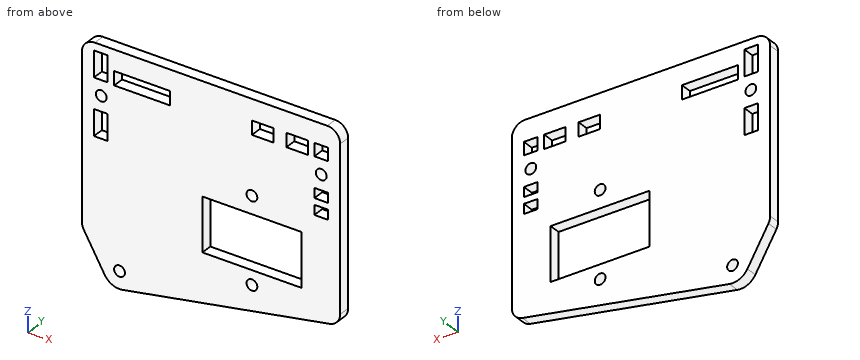
```python
from build123d import *
from build123d.topology import SkipClean

# Parameters (mm, degrees)
SKETCH1_R           = 1.25
SKETCH1_W           = 3.194492506
SKETCH1_H           = 3.000146449
SKETCH1_W_2         = 3.194434014
SKETCH1_H_2         = 6.000288014
SKETCH1_H_3         = 6.000224533
SKETCH1_W_3         = 4.990971694
SKETCH1_H_4         = 3.200091917
SKETCH1_W_4         = 4.991186163
SKETCH1_W_5         = 22.959409558
SKETCH1_H_5         = 12.40053533
BOSS_EXTRUDE1_DEPTH = 2.646066576


with BuildPart() as part:
    # Sketch1 → Boss-Extrude1 (new body)
    with SkipClean():  # the faces are left unmerged after this step: merging them gives an invalid solid
        with BuildSketch(Plane(origin=(0, 0, 0), x_dir=(1, 0, 0), z_dir=(0, 1, 0))):
            with BuildLine():
                Line((25.442900716, -27.532431428), (-28.456084878, -27.532431428))
                ThreePointArc((-28.456084878, -27.532431428), (-30.577373887, -26.653764751), (-31.456040564, -24.532475742))
                Line((-31.456040564, -24.532475742), (-31.456040564, 13.269326446))
                ThreePointArc((-31.456040564, 13.269326446), (-31.352979308, 14.049412081), (-31.050867612, 14.775968165))
                Line((-31.050867612, 14.775968165), (-26.174789125, 23.186205164))
                ThreePointArc((-26.174789125, 23.186205164), (-24.390968499, 24.809261571), (-21.997773241, 25.107497345))
                Line((-21.997773241, 25.107497345), (25.983223234, 16.219991273))
                ThreePointArc((25.983223234, 16.219991273), (27.743957441, 15.188191581), (28.437804204, 13.268980227))
                Line((28.437804204, 13.268980227), (28.437609204, -24.537738386))
                ThreePointArc((28.437609204, -24.537738386), (27.560473935, -26.65530708), (25.442900716, -27.532431428))
            make_face()
            with Locations(Location((-22.724218332, 21.185636807, 0), (0, 0, 270))):
                Circle(SKETCH1_R, mode=Mode.SUBTRACT)
            with Locations(Location((-26.963965218, -16.232064957, 0), (0, 0, 270))):
                Circle(SKETCH1_R, mode=Mode.SUBTRACT)
            with Locations(Location((7.974006473, 13.76898446, 0), (0, 0, 270))):
                Circle(SKETCH1_R, mode=Mode.SUBTRACT)
            with Locations(Location((7.974006472, -6.031549942, 0), (0, 0, 270))):
                Circle(SKETCH1_R, mode=Mode.SUBTRACT)
            with Locations(Location((24.045515173, -16.23206496, 0), (0, 0, 270))):
                Circle(SKETCH1_R, mode=Mode.SUBTRACT)
            Polygon((22.448181182, -10.478708085), (22.448181182, -10.484914569), (22.448181182, -12.731920553), (25.642673688, -12.731920553), (25.642673688, -10.478708085), align=None, mode=Mode.SUBTRACT)
            with Locations((24.045427435, -21.232282591)):
                Rectangle(SKETCH1_W, SKETCH1_H, mode=Mode.SUBTRACT)
            with Locations((-27.063830275, -9.731776544)):
                Rectangle(SKETCH1_W_2, SKETCH1_H_2, mode=Mode.SUBTRACT)
            with Locations((-27.063830276, -22.732321631)):
                Rectangle(SKETCH1_W_2, SKETCH1_H_3, mode=Mode.SUBTRACT)
            with Locations((18.446511119, -21.132309856)):
                Rectangle(SKETCH1_W_3, SKETCH1_H_4, mode=Mode.SUBTRACT)
            with Locations((10.460708795, -21.132309856)):
                Rectangle(SKETCH1_W_4, SKETCH1_H_4, mode=Mode.SUBTRACT)
            Polygon((-10.993335433, -19.532644781), (-10.993335433, -19.566758469), (-23.970138696, -19.566758469), (-23.970138696, -22.766982231), (-10.993335433, -22.766982231), align=None, mode=Mode.SUBTRACT)
            with Locations((7.974006472, 4.268713184)):
                Rectangle(SKETCH1_W_5, SKETCH1_H_5, mode=Mode.SUBTRACT)
            Polygon((25.642673689, -6.725489536), (25.642673689, -6.731632539), (22.448181183, -6.731632539), (22.448181183, -8.978702004), (25.642673689, -8.978702004), align=None, mode=Mode.SUBTRACT)
        extrude(amount=BOSS_EXTRUDE1_DEPTH)
    add(part.part.scale(1), mode=Mode.REPLACE)  # the faces are merged on a copy


solid = part.part
```
Geometry: final body of the model. Coordinates: model frame, mm. Coordinates: 2 decimals unless noted, no trailing zeros. Loops run counter-clockwise (first coordinate to the right, second up) from the corner with the lowest first, then second, coordinate; pieces in that order, holes last. Notation, with made-up numbers: (-26, 10) -> (14, 10) arc R23 cw to (14, 45) -> close; hole circle Ø1 at (-12, 50.5). An arc over 180 degrees is marked (long way). Use a Markdown table: item, result. Add a question column.
(1) Pin query (flat end, axial travel): pin 1 Ø3 at (x, z) = (-26.96, 16.23) entering from -Y; pin 2 Ø1.3 at (x, y) = (24, 2) entering from -Z. Return the tip coordinate at first contact, or that it passes through.
(2) Section query A-A, the plane z = -4. Return loops of the section in (x, y).
(3) Section query B-B, the plane x = -13.5. Return loops of the section in (y, z), plus the area to 3 significant figures.
(4) Section query D-D, the plane z = 16.5. Return loops of the section in (x, y), plus the area to 3 significant figures.
(5) Section query C-C, the plane x = 11. Return loops of the section in (y, z), plus the area to 3 significant figures.
(6) Line query: line 1 along X through (y, z) = (2.1, 22); line 2 along X through (y, z) = (0.15, 1); line 3 along Z through (x, y) = (-23, 2.1). Output: solid intervals per line, ascending.
Answer:
| question | item | result |
|---|---|---|
| 1 | pin 1 | stops at y = 0 |
| 1 | pin 2 | stops at z = -16.71 |
| 2 | outline | (-31.46, 0) -> (-3.51, 0) -> (-3.51, 2.65) -> (-31.46, 2.65) -> close; (19.45, 0) -> (28.44, 0) -> (28.44, 2.65) -> (19.45, 2.65) -> close |
| 3 | outline | (0, -23.53) -> (2.65, -23.53) -> (2.65, 19.57) -> (0, 19.57) -> close; (0, 22.77) -> (2.65, 22.77) -> (2.65, 27.53) -> (0, 27.53) -> close |
| 3 | area | 127 mm^2 |
| 4 | outline | (-31.46, 0) -> (-28.18, 0) -> (-28.18, 2.65) -> (-31.46, 2.65) -> close; (-25.74, 0) -> (22.82, 0) -> (22.82, 2.65) -> (-25.74, 2.65) -> close; (25.27, 0) -> (28.44, 0) -> (28.44, 2.65) -> (25.27, 2.65) -> close |
| 4 | area | 146 mm^2 |
| 5 | outline | (0, -19) -> (2.65, -19) -> (2.65, -10.47) -> (0, -10.47) -> close; (0, 1.93) -> (2.65, 1.93) -> (2.65, 19.53) -> (0, 19.53) -> close; (0, 22.73) -> (2.65, 22.73) -> (2.65, 27.53) -> (0, 27.53) -> close |
| 5 | area | 81.8 mm^2 |
| 6 | line 1 | x = -31.46 to -28.66, -25.47 to -23.97, -10.99 to 7.97, 12.96 to 15.95, 20.94 to 22.45, 25.64 to 28.44 |
| 6 | line 2 | x = -31.46 to -3.51, 19.45 to 28.44 |
| 6 | line 3 | z = -25.16 to -22.4, -19.97 to 19.57, 22.77 to 27.53 |
